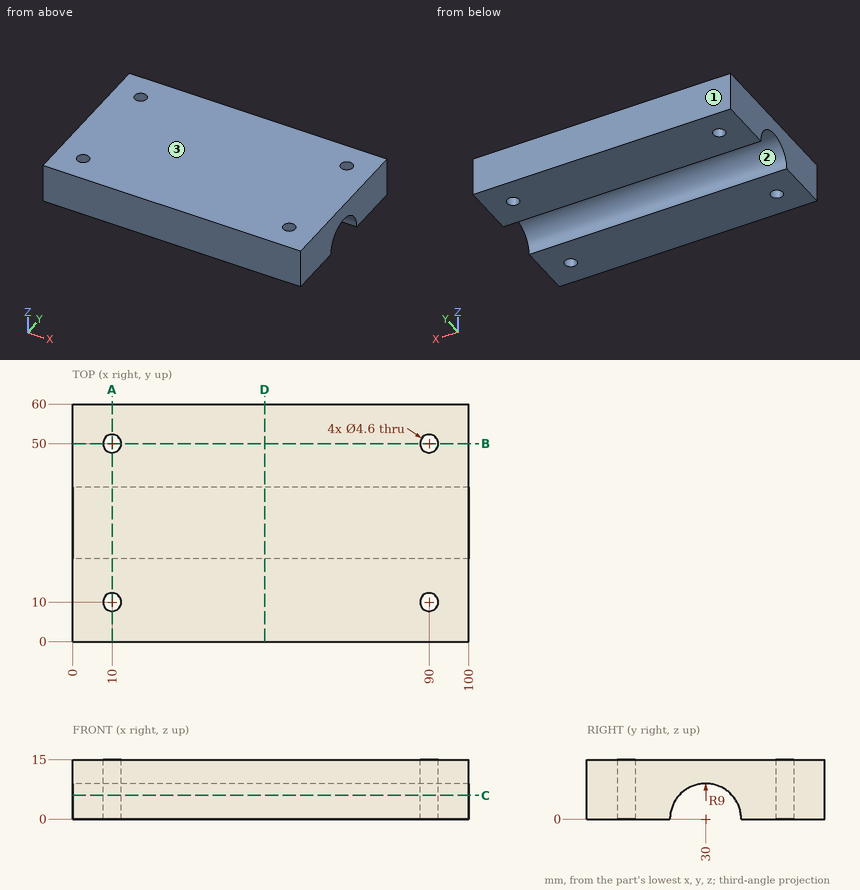
Part print with two shaded views. Sizes in mm from the minimum x, y, z corner. Round coordinates to 2 decimals unless told otherwise and drop trailing zeros. Loops run counter-clockwise (first coordinate to the right, second up) from the corner with the lowest first, then second, coordinate; pieces in that order, holes last.
Item 1: Two-plate mould, pull along Y, no slides. Class the marked faces 1, 2 and 3: released by +Y, released by -Y, zero draft, split by the parting line, or undercut.
Item 2: Saw through at A-A (x = 10). List the corners of the cut face in (y, z), then the cut area to 3 significant figures.
Item 3: Pin check, flat tip, straight feed: P1, Ø4, axis at x = 10, y = 10, coming from the -Z side. Stop position of the tip, or through.
Item 4: Saw through at C-C (z = 6). List the corners of the cut face in (x, y).
Item 5: Saw through at D-D (x = 48.5). List the corners of the cut face in (y, z), then the cut area to 3 significant figures.
Item 6: Drill centre lines: line 1 along Y through (x, z) = (90, 9.75); line 2 along Y through (x, z) = (10, 3.75); line 3 along Y through (x, z) = (33, 1.25). Where is each one in solid material? Low to high.
Item 7: Saw through at B-B (y = 50). List the corners of the cut face in (x, z), then the cut area to 3 significant figures.
Worked answers:
1. face 1: released by +Y
1. face 2: undercut
1. face 3: zero draft
2. outline: (0, 0) - (7.7, 0) - (7.7, 15) - (0, 15) - close; (12.3, 0) - (21, 0) arc R9 cw to (39, 0) - (47.7, 0) - (47.7, 15) - (12.3, 15) - close; (52.3, 0) - (60, 0) - (60, 15) - (52.3, 15) - close
2. area: 635 mm2
3. P1: passes through
4. outline: (0, 0) - (100, 0) - (100, 23.29) - (0, 23.29) - close; (0, 36.71) - (100, 36.71) - (100, 60) - (0, 60) - close; hole circle Ø4.6 at (10, 10); hole circle Ø4.6 at (10, 50); hole circle Ø4.6 at (90, 10); hole circle Ø4.6 at (90, 50)
5. outline: (0, 0) - (21, 0) arc R9 cw to (39, 0) - (60, 0) - (60, 15) - (0, 15) - close
5. area: 773 mm2
6. line 1: y = 0 to 7.7, 12.3 to 47.7, 52.3 to 60
6. line 2: y = 0 to 7.7, 12.3 to 21.82, 38.18 to 47.7, 52.3 to 60
6. line 3: y = 0 to 21.09, 38.91 to 60
7. outline: (0, 0) - (7.7, 0) - (7.7, 15) - (0, 15) - close; (12.3, 0) - (87.7, 0) - (87.7, 15) - (12.3, 15) - close; (92.3, 0) - (100, 0) - (100, 15) - (92.3, 15) - close
7. area: 1,360 mm2
